from build123d import *

# Parameters (mm, degrees)
BOSS_EXTRUDE1_DEPTH       = 10
CUT_EXTRUDE1_DEPTH        = 10
CUT_EXTRUDE1_DEPTH_BACK   = 10
SKETCH2_R                 = 5
CUT_SWEEP1_PITCH          = 4
CUT_SWEEP1_HEIGHT         = 10
CUT_SWEEP1_RADIUS         = 5
EXTRUDE_THIN2_DEPTH       = 10
BODY_MOVE_COPY1_ANGLE     = 2
SKETCH10_W                = 58.079037791
SKETCH10_H                = 9.197874715
BOSS_EXTRUDE2_DEPTH       = 10
SKETCH21_R                = 37.93035277
BOSS_EXTRUDE11_DEPTH      = 4
CUT_EXTRUDE5_DEPTH        = 4
CUT_EXTRUDE5_DEPTH_BACK   = 4
SKETCH22_R                = 12.7
CUT_EXTRUDE6_DEPTH        = 4
CUT_EXTRUDE6_DEPTH_BACK   = 4
SKETCH23_R                = 4.76
CUT_EXTRUDE7_DEPTH        = 4
CUT_EXTRUDE7_DEPTH_BACK   = 4
SKETCH24_R                = 4.76
BOSS_EXTRUDE13_DEPTH      = 1
BOSS_EXTRUDE13_DEPTH_BACK = 7.87
SKETCH27_R                = 6.76
CUT_EXTRUDE12_DEPTH       = 1
CUT_EXTRUDE12_DEPTH_BACK  = 7.87
SKETCH28_R                = 4.76
BOSS_EXTRUDE14_DEPTH      = 1
BOSS_EXTRUDE14_DEPTH_BACK = 7.87
SKETCH29_R                = 6.76
CUT_EXTRUDE13_DEPTH       = 1
CUT_EXTRUDE13_DEPTH_BACK  = 7.87
SKETCH30_R                = 4.585303289
SKETCH20_W                = 8.892243229
SKETCH20_H                = 10.060161684
BOSS_EXTRUDE15_DEPTH      = 10
SKETCH19_R                = 15
BOSS_EXTRUDE16_DEPTH      = 10
CUT_EXTRUDE14_DEPTH       = 10
CUT_EXTRUDE14_DEPTH_BACK  = 10
SKETCH31_R                = 12.7


with BuildPart() as part:
    # Sketch1 → Boss-Extrude1 (new body)
    with BuildSketch(Plane.XY):
        Polygon((-8.167579482, -4.315550803), (-0.346413115, -9.231106721), (7.821166368, -4.915555918), (8.167579482, 4.315550803), (0.346413115, 9.231106721), (-7.821166368, 4.915555918), align=None)
    extrude(amount=BOSS_EXTRUDE1_DEPTH)

    # Sketch2 → Cut-Extrude1 (cut, two sides: drawn at the far end of the back side and taken through both)
    with BuildSketch(Plane.XY.offset(-CUT_EXTRUDE1_DEPTH_BACK)):
        Circle(SKETCH2_R)
    extrude(amount=CUT_EXTRUDE1_DEPTH + CUT_EXTRUDE1_DEPTH_BACK, mode=Mode.SUBTRACT)

    # Cut-Sweep1: sweep along a helix
    with BuildLine() as cut_sweep1_path:
        Helix(CUT_SWEEP1_PITCH, CUT_SWEEP1_HEIGHT, CUT_SWEEP1_RADIUS, center=(0, 0, 0), direction=(0, 0, 1), lefthand=True)
    # Sketch4 → Cut-Sweep1 (sweep, cut)
    with BuildSketch(Plane.XY):
        Polygon((5.337109255, 0), (4.831445373, 0.291945178), (4.831445373, -0.291945178), align=None)
    sweep(path=cut_sweep1_path.line, is_frenet=True, mode=Mode.SUBTRACT)

    # Sketch6 → Extrude-Thin2 (add)
    with BuildSketch(Plane.XY):
        Polygon((-7.821166368, 4.915555918), (-8.167579482, -4.315550803), (-18.160545639, -3.940547606), (-17.814132524, 5.290559115), align=None)
    extrude(amount=EXTRUDE_THIN2_DEPTH)


with BuildPart() as part_1:
    # Body-Move/Copy1: moved
    add(part.part.rotate(Axis((-4.996483078, 0, 0), (0, 0, 1)), BODY_MOVE_COPY1_ANGLE))

    # Sketch10 → Boss-Extrude2 (add)
    with BuildSketch(Plane.XY):
        with Locations((-47.030481105, 0.241069377)):
            Rectangle(SKETCH10_W, SKETCH10_H)
    extrude(amount=BOSS_EXTRUDE2_DEPTH)

    # Sketch21 → Boss-Extrude11 (add)
    with BuildSketch(Plane.XY):
        with Locations((-113.262670717, 0)):
            Circle(SKETCH21_R)
    extrude(amount=BOSS_EXTRUDE11_DEPTH)

    # Sketch22 → Cut-Extrude5 (cut, two sides: drawn at the far end of the back side and taken through both)
    with BuildSketch(Plane.XY.offset(-CUT_EXTRUDE5_DEPTH_BACK)):
        with Locations((-113.262670717, 0)):
            Circle(SKETCH22_R)
    extrude(amount=CUT_EXTRUDE5_DEPTH + CUT_EXTRUDE5_DEPTH_BACK, mode=Mode.SUBTRACT)

    # Sketch23 → Cut-Extrude6 (cut, two sides: drawn at the far end of the back side and taken through both)
    with BuildSketch(Plane.XY.offset(-CUT_EXTRUDE6_DEPTH_BACK)):
        with Locations((-112.966619713, 25.4)):
            Circle(SKETCH23_R)
    extrude(amount=CUT_EXTRUDE6_DEPTH + CUT_EXTRUDE6_DEPTH_BACK, mode=Mode.SUBTRACT)

    # Sketch24 → Cut-Extrude7 (cut, two sides: drawn at the far end of the back side and taken through both)
    with BuildSketch(Plane.XY.offset(-CUT_EXTRUDE7_DEPTH_BACK)):
        with Locations((-112.471115727, -25.4)):
            Circle(SKETCH24_R)
    extrude(amount=CUT_EXTRUDE7_DEPTH + CUT_EXTRUDE7_DEPTH_BACK, mode=Mode.SUBTRACT)

    # Sketch27 → Boss-Extrude13 (add, two sides: drawn at the far end of the back side and taken through both)
    with BuildSketch(Plane.XY.offset(-BOSS_EXTRUDE13_DEPTH_BACK)):
        with Locations((-112.966619713, 25.4)):
            Circle(SKETCH27_R)
    extrude(amount=BOSS_EXTRUDE13_DEPTH + BOSS_EXTRUDE13_DEPTH_BACK)

    # Sketch28 → Cut-Extrude12 (cut, two sides: drawn at the far end of the back side and taken through both)
    with BuildSketch(Plane.XY.offset(-CUT_EXTRUDE12_DEPTH_BACK)):
        with Locations((-112.966619713, 25.4)):
            Circle(SKETCH28_R)
    extrude(amount=CUT_EXTRUDE12_DEPTH + CUT_EXTRUDE12_DEPTH_BACK, mode=Mode.SUBTRACT)

    # Sketch29 → Boss-Extrude14 (add, two sides: drawn at the far end of the back side and taken through both)
    with BuildSketch(Plane(origin=(-24.725624919, 0.221889436, 0), x_dir=(1, 0, 0), z_dir=(0, 0, 1)).offset(-BOSS_EXTRUDE14_DEPTH_BACK)):
        with Locations((-87.745490808, -25.657760722)):
            Circle(SKETCH29_R)
    extrude(amount=BOSS_EXTRUDE14_DEPTH + BOSS_EXTRUDE14_DEPTH_BACK)

    # Sketch30 → Cut-Extrude13 (cut, two sides: drawn at the far end of the back side and taken through both)
    with BuildSketch(Plane.XY.offset(-CUT_EXTRUDE13_DEPTH_BACK)):
        with Locations(Location((-112.583618689, -25.142193243, 0), (0, 0, 166.546290498))):
            Circle(SKETCH30_R)
    extrude(amount=CUT_EXTRUDE13_DEPTH + CUT_EXTRUDE13_DEPTH_BACK, mode=Mode.SUBTRACT)

    # Sketch20 → Boss-Extrude15 (add)
    with BuildSketch(Plane.XY):
        with Locations((-152.872413964, 0)):
            Rectangle(SKETCH20_W, SKETCH20_H)
    extrude(amount=BOSS_EXTRUDE15_DEPTH)

    # Sketch19 → Boss-Extrude16 (add)
    with BuildSketch(Plane.XY):
        with Locations((-171.45, 0)):
            Circle(SKETCH19_R)
    extrude(amount=BOSS_EXTRUDE16_DEPTH)

    # Sketch31 → Cut-Extrude14 (cut, two sides: drawn at the far end of the back side and taken through both)
    with BuildSketch(Plane.XY.offset(-CUT_EXTRUDE14_DEPTH_BACK)):
        with Locations((-171.028613762, 0)):
            Circle(SKETCH31_R)
    extrude(amount=CUT_EXTRUDE14_DEPTH + CUT_EXTRUDE14_DEPTH_BACK, mode=Mode.SUBTRACT)


solid = part_1.part
Here's how the part is built. I have some questions about the finished solid (model axes, mm). A direction names the side the tool comes from. Coordinates: 2 decimals unless noted, no trailing zeros. Loops run counter-clockwise (first coordinate to the right, second up) from the corner with the lowest first, then second, coordinate; pieces in that order, holes last.
1. For P1, Ø3, axis at y = 22.5, z = 0.5, coming from the -X side; P2, Ø3, axis at x = -33, z = 2.5, coming from the +Y side; P3, Ø5, axis at x = -42, z = 4, coming from the -Y side, each with a flat end and sliding along its axis, tell me the tip position at first contact or that it passes through.
2. I need wall thicknesses on L1, parallel to X at y = 0, z = 1.3; L2, parallel to X at y = 0, z = 6.75; L3, parallel to Y at x = -152, z = 6.75. Which ranges of each line are inside material? Lowest first, please.
3. Imagine slicing it at A-A, the plane y = 25.4. Please give me the cut outline in (x, z).
4. Imagine slicing it at C-C, the plane x = -171.45. Please give me the cut outline in (y, z), and give its area (3 significant figures).
5. For faces 4 (the flat face through (-76.07, 0, 7)), 5 (the flat face through (-153, 5.03, 5)), 6 (the flat face through (-4.08, -6.71, 4.93)), which set-ups out of +Z, -Z, +X, -X, +Y, -Y let a thin tool reach every point of the face, with its end or its side?
6. Imagine slicing it at B-B, the plane y = -11. Please give me the cut outline in (x, z), and give its area (3 significant figures).
7. If we mould it in two halves opening along X, with no side actions, what happens to faces 1 (the flat face through (-148.426, 0, 7)), 2 (the flat face through (4.07, 7.06, 4.93)), 3 (the flat face through (-113, -30, -7.87))? For each: pulls with the +X half, pulls with the -X half, needs draft (parallel to the pull), parting line crosses it, or undercut.
Taken from the geometry:
1. P1: stops at x = -144.85
1. P2: stops at y = 4.84
1. P3: stops at y = -4.36
2. L1: x = -186.45 to -183.73, -158.33 to -125.96, -100.56 to -5, 4.99 to 8
2. L2: x = -186.45 to -183.73, -158.33 to -148.43, -76.07 to -5, 4.99 to 8
2. L3: y = -5.03 to 5.03
3. outline: (-141.43, 0) - (-119.73, 0) - (-119.73, -7.87) - (-117.73, -7.87) - (-117.73, 4) - (-141.43, 4) - close; (-108.21, -7.87) - (-106.21, -7.87) - (-106.21, 0) - (-85.09, 0) - (-85.09, 4) - (-108.21, 4) - close
4. outline: (-15, 0) - (-12.69, 0) - (-12.69, 10) - (-15, 10) - close; (12.69, 0) - (15, 0) - (15, 10) - (12.69, 10) - close
4. area: 46.1 mm2
5. face 4: +Z, +Y, -Y
5. face 5: +Z, +Y
5. face 6: +Z, -Z, -Y
6. outline: (-181.65, 0) - (-177.38, 0) - (-177.38, 10) - (-181.65, 10) - close; (-164.68, 0) - (-161.25, 0) - (-161.25, 10) - (-164.68, 10) - close; (-149.56, 0) - (-119.61, 0) - (-119.61, 4) - (-149.56, 4) - close; (-106.92, 0) - (-76.96, 0) - (-76.96, 4) - (-106.92, 4) - close
6. area: 317 mm2
7. face 1: undercut
7. face 2: pulls with the +X half
7. face 3: needs draft
